Check sheet for the modelled part. Datum: model origin and axes. Units: mm. Face numbers are marked on the shaded views. A direction names the side the tool comes from. Coordinates: 2 decimals unless noted, no trailing zeros. Order: outer loops, then holes, each group sorted by start corner. A loop starts at its lowest first (then second) coordinate and runs counter-clockwise, first axis right, second up.
1. Cross-section at D-D (x = 8). Enter the section's corners in (y, z).
2. Cross-section at B-B (x = -26). Enter the section's corners in (y, z).
3. Cross-section at A-A (y = 0). Enter the section's corners in (x, z).
4. Cross-section at C-C (z = 26.5). Enter the section's corners in (x, y), then the cut area to 3 significant figures.
5. Thickness scan on line 1 (Y direction, x = 0, z = 19.25); line 2 (X direction, y = -10.5, z = 18.25); line 3 (Y direction, x = 8, z = 15.25). Record the ranges inside material, lowest first.
6. Gauge pin test, flat ends, axial feed: pin 1 Ø6 at (y, z) = (-7, 19) entering from -X; pin 2 Ø16 at (y, z) = (-4.5, 19.5) entering from +X; pin 3 Ø3 at (y, z) = (-17.5, 20.5) entering from +X. Record the tip position at first contact, or that the pin passes through.
7. Set-up check for the marked faces 1 and 2: record each of +Z, -Z, +X, -X, +Y, -Y from which the full face is reachable in a straight line by a thin tool's end or side.
8. Draft check along Z on the marked faces 3, 4 and 5. Enter one of: released by +Z, released by -Z, zero draft, split by the parting line, or undercut.
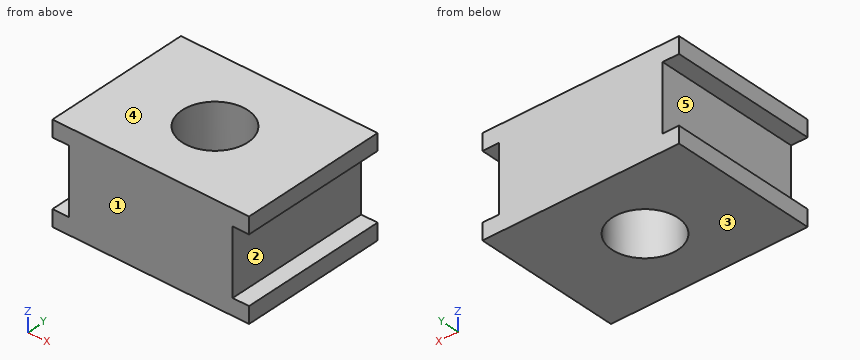
```python
from build123d import *

# Parameters (mm, degrees)
SKETCH_1_W          = 60
SKETCH_1_H          = 45
EXTRUDE_1_DEPTH     = 30
SKETCH_2_W          = 15
SKETCH_2_H          = 20
CUT_EXTRUDE_1_DEPTH = 80
SKETCH_3_R          = 10
CUT_EXTRUDE_2_DEPTH = 80


with BuildPart() as part:
    # 草图1 → 凸台-拉伸1 (new body)
    with BuildSketch(Plane.XY):
        Rectangle(SKETCH_1_W, SKETCH_1_H)
    extrude(amount=EXTRUDE_1_DEPTH)

    # 草图2 → 切除-拉伸1 (cut)
    with BuildSketch(Plane(origin=(0, 22.5, 0), x_dir=(1, 0, 0), z_dir=(0, 1, 0))):
        with Locations((-32.5, -15)):
            Rectangle(SKETCH_2_W, SKETCH_2_H)
        with Locations((32.5, -15)):
            Rectangle(SKETCH_2_W, SKETCH_2_H)
    extrude(amount=-CUT_EXTRUDE_1_DEPTH, mode=Mode.SUBTRACT)

    # 草图3 → 切除-拉伸2 (cut)
    with BuildSketch(Plane.XY.offset(30)):
        Circle(SKETCH_3_R)
    extrude(amount=-CUT_EXTRUDE_2_DEPTH, mode=Mode.SUBTRACT)


solid = part.part
```
Data:
1. outline: (-22.5, 0) - (-6, 0) - (-6, 30) - (-22.5, 30) - close; (6, 0) - (22.5, 0) - (22.5, 30) - (6, 30) - close
2. outline: (-22.5, 0) - (22.5, 0) - (22.5, 5) - (-22.5, 5) - close; (-22.5, 25) - (22.5, 25) - (22.5, 30) - (-22.5, 30) - close
3. outline: (-30, 0) - (-10, 0) - (-10, 30) - (-30, 30) - (-30, 25) - (-25, 25) - (-25, 5) - (-30, 5) - close; (10, 0) - (30, 0) - (30, 5) - (25, 5) - (25, 25) - (30, 25) - (30, 30) - (10, 30) - close
4. outline: (-30, -22.5) - (30, -22.5) - (30, 22.5) - (-30, 22.5) - close; hole circle Ø20 at (0, 0)
4. area: 2,390 mm2
5. line 1: y = -22.5 to -10, 10 to 22.5
5. line 2: x = -25 to 25
5. line 3: y = -22.5 to -6, 6 to 22.5
6. pin 1: stops at x = -25
6. pin 2: stops at x = 30
6. pin 3: stops at x = 25
7. face 1: +Z, -Z, +X, -X, -Y
7. face 2: +X, +Y, -Y
8. face 3: released by -Z
8. face 4: released by +Z
8. face 5: undercut
